```python
from build123d import *

# Parameters (mm, degrees)
BOSS_EXTRUDE1_OUTLINE_R = 6.35
BOSS_EXTRUDE1_DEPTH     = 132.09778


# Read off the part's stored shape, not the designer's step: Boss-Extrude1
with BuildPart() as part:
    # Boss-Extrude1 outline → Boss-Extrude1 (new body)
    with BuildSketch(Plane.XY.offset(-22.86)):
        Circle(BOSS_EXTRUDE1_OUTLINE_R)
    extrude(amount=BOSS_EXTRUDE1_DEPTH)


solid = part.part
```
Work out the finished part from the listing and answer in its coordinate system (mm). Coordinates: 2 decimals unless noted, no trailing zeros. Loops run counter-clockwise (first coordinate to the right, second up) from the corner with the lowest first, then second, coordinate; pieces in that order, holes last. Notation, with made-up numbers: M 82.25,-36.5 L 127.25,-36.5 A25 cw 127.25,-13.5 Z; hole C -37.75,-36.5 d4. An arc over 180 degrees is marked long. Use CSV: the item, a comma, the result in double quotes. Start each with the question number.
(1) Find section B-B, the plane y = -1.25. Give the vertices of the cut face in (x, z), then the cut area to 3 significant figures.
(2) Given pin 1 Ø3 at (x, z) = (-3.5, 61.5) entering from +Y; pin 2 Ø1.5 at (x, z) = (-4.5, 4) entering from -Y; pin 3 Ø5 at (y, z) = (-2, 66) entering from -X, each flat-ended and moving along its own axis, determine where each tip first touches the part or whether it passes through.
(3) Find section C-C, the plane x = -3.5. Give the vertices of the cut face in (y, z).
(4) Consider line 1 (Y direction, x = 0.5, z = 31.5); line 2 (Y direction, x = 1.5, z = 30). Determine where each line is inside the solid, lowest interval first.
(5) Find section A-A, the plane z = -12.5. Give the vertices of the cut face in (x, y).
Recorded:
1,outline,"M -6.23,-22.86 L 6.23,-22.86 L 6.23,109.24 L -6.23,109.24 Z"
1,area,"1,640 mm^2"
2,pin 1,"stops at y = 6.03"
2,pin 2,"stops at y = -5.12"
2,pin 3,"stops at x = -6.35"
3,outline,"M -5.3,-22.86 L 5.3,-22.86 L 5.3,109.24 L -5.3,109.24 Z"
4,line 1,"y = -6.33 to 6.33"
4,line 2,"y = -6.17 to 6.17"
5,outline,"C 0,0 d12.7"
